Design review of the part built by this model. Coordinates are the model's own, in mm. Face numbers are marked on the shaded views. A direction names the side the tool comes from. Round coordinates to 2 decimals unless told otherwise and drop trailing zeros. Write each loop counter-clockwise with the first axis right and the second up, starting at its lowest first coordinate (ties: lowest second). Pieces come first, ordered by that corner, then holes. Notation, with made-up numbers: M -18.75,1.5 L -14.75,1.5 A6 cw -14.75,5.5 Z; hole C 49,43 d3. An arc over 180 degrees is marked long. Use CSV: the item, a comma, the result in double quotes.
from build123d import *

# Parameters (mm, degrees)
BOSS_EXTRUDE1_DEPTH = 22
FILLET10_R          = 2
FILLET11_R          = 2
SKETCH4_W           = 40
SKETCH4_H           = 18.455921649
CUT_EXTRUDE1_DEPTH  = 30
FILLET12_R          = 2


with BuildPart() as part:
    # Sketch2 → Boss-Extrude1 (new body)
    with BuildSketch(Plane.XY):
        Polygon((-70.922010647, 6.21881141), (23.946585559, 6.21881141), (29.020925711, 4.371902636), (28.507895496, 2.962363705), (22.467605346, 5.160849526), (-64.922010647, 5.160849526), (-70.922010647, 6.060990271), align=None)
    extrude(amount=BOSS_EXTRUDE1_DEPTH)

    # Fillet10
    fillet10_edges = [part.edges().sort_by_distance(p)[0] for p in [
        (28.764410604, 3.667133171, 22),
        (28.764410604, 3.667133171, 0),
    ]]
    fillet(fillet10_edges, radius=FILLET10_R)

    # Fillet11
    fillet11_edges = [part.edges().sort_by_distance(p)[0] for p in [
        (23.946585559, 6.21881141, 11),
    ]]
    fillet(fillet11_edges, radius=FILLET11_R)

    # Sketch4 → Cut-Extrude1 (cut)
    with BuildSketch(Plane.XZ.offset(-5.160849526)):
        with Locations((-34.922010647, 20.227960825)):
            Rectangle(SKETCH4_W, SKETCH4_H)
        with BuildLine():
            Line((-59.68856271, 8.67422642), (-59.68856271, 17))
            ThreePointArc((-59.68856271, 17), (-60.922010647, 18.233447938), (-62.155458585, 17))
            Line((-62.155458585, 17), (-62.155458585, 8.67422642))
            ThreePointArc((-62.155458585, 8.67422642), (-60.922010647, 7.440778483), (-59.68856271, 8.67422642))
        make_face()
        with BuildLine():
            Line((-7.739956374, 8.67422642), (-7.739956374, 17))
            ThreePointArc((-7.739956374, 17), (-8.922010647, 18.182054274), (-10.104064921, 17))
            Line((-10.104064921, 17), (-10.104064921, 8.67422642))
            ThreePointArc((-10.104064921, 8.67422642), (-8.922010647, 7.492172147), (-7.739956374, 8.67422642))
        make_face()
    extrude(amount=-CUT_EXTRUDE1_DEPTH, mode=Mode.SUBTRACT)

    # Fillet12
    fillet12_edges = [part.edges().sort_by_distance(p)[0] for p in [
        (-14.922010647, 5.689830468, 11),
        (-54.922010647, 5.689830468, 11),
    ]]
    fillet(fillet12_edges, radius=FILLET12_R)


solid = part.part
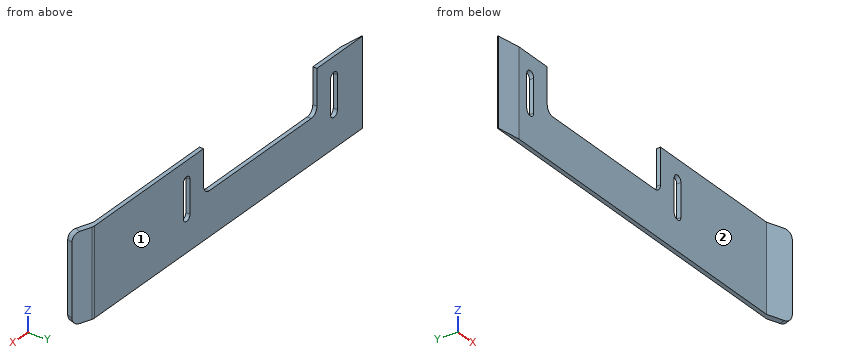
1) Add section A-A on z = 9.75. Write out the cut boundary in (x, y), then the cut area to 3 significant figures.
Answers:
outline,"M -70.92,6.06 L -64.92,5.16 L -62.16,5.16 L -62.16,6.22 L -70.92,6.22 Z; M -59.69,5.16 L -10.1,5.16 L -10.1,6.22 L -59.69,6.22 Z; M -7.74,5.16 L 22.47,5.16 L 28.51,2.96 L 29.02,4.37 L 24.28,6.1 A2 ccw 23.59,6.22 L -7.74,6.22 Z"
area,"101 mm²"
2) Wall thickness on line 1 along Y through (x, z) = (14, 19.5); line 2 along Y through (x, z) = (23.5, 5.5): over which ranges is each line inside the solid? List them lowest first. Write a range as [from, to].
Answers:
line 1,"[5.16, 6.22]"
line 2,"[4.79, 6.22]"
3) For pin 1 Ø4 at (x, z) = (4, 7) entering from -Y; pin 2 Ø2 at (x, z) = (-46, 13) entering from +Y; pin 3 Ø0.5 at (x, y) = (-41.5, 6) entering from +Z, all flat-tipped, find the tip position at first contact; note any pin that passes through.
Answers:
pin 1,"y = 5.16"
pin 2,"through"
pin 3,"z = 11"
4) Add section B-B on x = -11.5. Write out the cut boundary in (y, z).
Answers:
outline,"M 5.16,0 L 6.22,0 L 6.22,22 L 5.16,22 Z"
5) Machinability: for the marked faces 1 and 2, which of the approach directions +Z, -Z, +X, -X, +Y, -Y give a long, thin tool a straight path to every point of the face, cutting with its end or side? Answer none if there is none.
Answers:
face 1,"+Z, -Z, +X, -X, +Y"
face 2,"+Z, -Z, -X, -Y"
